from build123d import *

# Parameters (mm, degrees)
F1_DEPTH = 25
F2_W     = 36.5
F2_H     = 7
F3_DEPTH = 1
F4_W     = 36.5
F4_H     = 7
F5_DEPTH = 1


with BuildPart() as f1:
    # F0 (on Top) → F1 (new body)
    with BuildSketch(Plane.XY):
        with BuildLine():
            ThreePointArc((19.203308, -7.914208), (8.453308, 2.835792), (19.203308, 13.585792))
            Line((19.203308, 13.585792), (19.203308, 16.585792))
            Line((19.203308, 16.585792), (-17.296692, 16.585792))
            Line((-17.296692, 16.585792), (-17.296692, 13.585792))
            ThreePointArc((-17.296692, 13.585792), (-9.695294, 10.43719), (-6.546692, 2.835792))
            ThreePointArc((-6.546692, 2.835792), (-9.695294, -4.765606), (-17.296692, -7.914208))
            Line((-17.296692, -7.914208), (-17.296692, -10.914208))
            Line((-17.296692, -10.914208), (19.203308, -10.914208))
            Line((19.203308, -10.914208), (19.203308, -7.914208))
        make_face()
    extrude(amount=F1_DEPTH)

    # F2 (on face) → F3 (cut)
    with BuildSketch(Plane.XZ.offset(10.914208)):
        with Locations((0.953308, 12.5)):
            Rectangle(F2_W, F2_H)
    extrude(amount=-F3_DEPTH, mode=Mode.SUBTRACT)

    # F4 (on face) → F5 (cut)
    with BuildSketch(Plane(origin=(0, 16.585792, 0), x_dir=(-1, 0, 0), z_dir=(0, 1, 0))):
        with Locations((-0.953308, 12.039038)):
            Rectangle(F4_W, F4_H)
    extrude(amount=-F5_DEPTH, mode=Mode.SUBTRACT)


solid = f1.part
Geometry check sheet. Reference: the model listing, model coordinates, mm. A direction names the side the tool comes from. Round coordinates to 2 decimals unless told otherwise and drop trailing zeros. Order: outer loops, then holes, each group sorted by start corner. A loop starts at its lowest first (then second) coordinate and runs counter-clockwise, first axis right, second up. Notation, with made-up numbers: M -13,53 L 14,53 A17 cw 14,69 Z; hole C 60,14 d1. An arc over 180 degrees is marked long. Write each question's results on one line, items separated by ' | '. Start each with the question number.
1. Set-up check for faces 1 (the face through (1, 16, 8.539)), 2 (the face through (-17.297, -9, 12)), 3 (the face through (0.7, -10.4, 9)): record each of +Z, -Z, +X, -X, +Y, -Y from which the full face is reachable in a straight line by a thin tool's end or side.
2. Cross-section at C-C on x = -4.5. Record the boundary of the cut face in (y, z).
3. Cross-section at A-A on x = 15. Record the boundary of the cut face in (y, z), plus the area to 3 significant figures.
4. Material ranges on L1, parallel to Y at x = -5.5, z = 8.75; L2, parallel to Y at x = -8.5, z = 6.5; L3, parallel to X at y = 3.25, z = 11, recorded low to high. Write a range as from..to.
5. Cross-section at B-B on z = 7.5. Record the boundary of the cut face in (x, y), plus the area to 3 significant figures.
6. Go/stop test with flat-tipped pins: P1, Ø5.5, axis at x = -8, z = 12.5, coming from the -Y side; P2, Ø4, axis at y = 6.5, z = 3.5, coming from the -X side. Record where each tip stops, or that it passes through.
7. Cross-section at D-D on y = 8. Record the boundary of the cut face in (x, z), plus the area to 3 significant figures.
8. Draft check along Z on faces 4 (the face through (1, 3, 0)), 5 (the face through (-17.297, 15, 12)), 6 (the face through (0.7, -10.4, 16)). Enter one of: pulls with the +Z half, pulls with the -Z half, needs draft (parallel to the pull), parting line crosses it, or undercut.
Resolved:
1) face 1: +X, -X, +Y | face 2: +Z, -Z, -X, +Y, -Y | face 3: +X, -X, -Y
2) outline: M -10.91,0 L 16.59,0 L 16.59,8.54 L 15.59,8.54 L 15.59,15.54 L 16.59,15.54 L 16.59,25 L -10.91,25 L -10.91,16 L -9.91,16 L -9.91,9 L -10.91,9 Z
3) outline: M -10.91,0 L -7.06,0 L -7.06,25 L -10.91,25 L -10.91,16 L -9.91,16 L -9.91,9 L -10.91,9 Z; M 12.73,0 L 16.59,0 L 16.59,8.54 L 15.59,8.54 L 15.59,15.54 L 16.59,15.54 L 16.59,25 L 12.73,25 Z | area: 179 mm2
4) L1: -10.91..15.59 | L2: -10.91..-3.34, 9.01..16.59 | L3: -6.55..8.46
5) outline: M -17.3,-10.91 L 19.2,-10.91 L 19.2,-7.91 A10.75 cw 19.2,13.59 L 19.2,16.59 L -17.3,16.59 L -17.3,13.59 A10.75 cw -17.3,-7.91 Z | area: 641 mm2
6) P1: y = -9.91 | P2: x = -8.16
7) outline: M -7.87,0 L 9.77,0 L 9.77,25 L -7.87,25 Z | area: 441 mm2
8) face 4: pulls with the -Z half | face 5: needs draft | face 6: undercut
